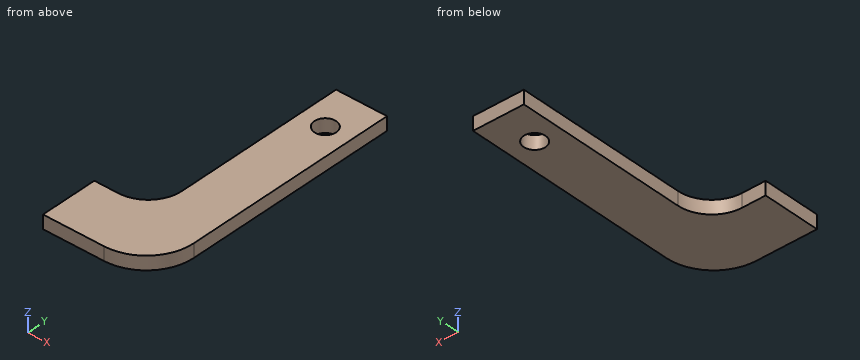
```python
from build123d import *

# Parameters (mm, degrees)
SKETCH_1_R      = 1.6
EXTRUDE_1_DEPTH = 2


with BuildPart() as part:
    # 草图1 → 凸台-拉伸1 (new body)
    with BuildSketch(Plane.XY):
        with BuildLine():
            Line((-7.738670695, -1.280966767), (-11.238670695, -1.280966767))
            Line((-11.238670695, -1.280966767), (-11.238670695, -9.780966767))
            Line((-11.238670695, -9.780966767), (-2.738670695, -9.780966767))
            Line((-2.738670695, -9.780966767), (-2.238670695, -9.780966767))
            ThreePointArc((-2.238670695, -9.780966767), (2.711076773, -7.730714236), (4.761329305, -2.780966767))
            Line((4.761329305, -2.780966767), (4.761329305, -1.280966767))
            Line((4.761329305, -1.280966767), (4.761329305, 29.219033233))
            Line((4.761329305, 29.219033233), (-2.738670695, 29.219033233))
            Line((-2.738670695, 29.219033233), (-2.738670695, 3.719033233))
            ThreePointArc((-2.738670695, 3.719033233), (-4.203136789, 0.183499327), (-7.738670695, -1.280966767))
        make_face()
        with Locations((1.011329305, 23.219033233)):
            Circle(SKETCH_1_R, mode=Mode.SUBTRACT)
    extrude(amount=EXTRUDE_1_DEPTH)


solid = part.part
```
Source: CAD feature listing. Evaluate the final solid. Frame: model axes, mm. Coordinates: 2 decimals unless noted, no trailing zeros. Loops run counter-clockwise (first coordinate to the right, second up) from the corner with the lowest first, then second, coordinate; pieces in that order, holes last. Notation, with made-up numbers: (58.5, 10) - (74.5, 10) arc R8 ccw to (74.5, 23) - close; hole circle Ø2 at (25, -10.75). An arc over 180 degrees is marked (long way). Answer as CSV lines item,"result".
1. Ray query, line 1 (Y direction, x = 0.5, z = 1.6); line 2 (Y direction, x = -2, z = 0.8); line 3 (Y direction, x = 1.5, z = 0.55). Return the intervals inside material, ascending.
Established:
line 1,"y = -9.22 to 21.7, 24.74 to 29.22"
line 2,"y = -9.78 to 29.22"
line 3,"y = -8.7 to 21.7, 24.74 to 29.22"
2. Section A-A (z = 0.85). Return loops of the section in (x, y).
Established:
outline,"(-11.24, -9.78) - (-2.24, -9.78) arc R7 ccw to (4.76, -2.78) - (4.76, 29.22) - (-2.74, 29.22) - (-2.74, 3.72) arc R5 cw to (-7.74, -1.28) - (-11.24, -1.28) - close; hole circle Ø3.2 at (1.01, 23.22)"
3. Section B-B (y = 11). Return loops of the section in (x, z).
Established:
outline,"(-2.74, 0) - (4.76, 0) - (4.76, 2) - (-2.74, 2) - close"
4. Contact query for flat-ended pins moving along their axis: pin 1 (2 mm diameter, centred on x = -5.5, y = 6.5, fed in from +Z); pin 2 (1 mm diameter, centred on y = 20, z = 1.5, fed in from -X); pin 3 (3.5 mm diameter, centred on x = 1.01, y = 23.22, fed in from -Z). Output: stop coordinate, or through.
Established:
pin 1,"passes through"
pin 2,"stops at x = -2.74"
pin 3,"stops at z = 0"
5. Section C-C (x = -9.5). Return loops of the section in (y, z), then the cut area to 3 significant figures.
Established:
outline,"(-9.78, 0) - (-1.28, 0) - (-1.28, 2) - (-9.78, 2) - close"
area,"17.0 mm2"
